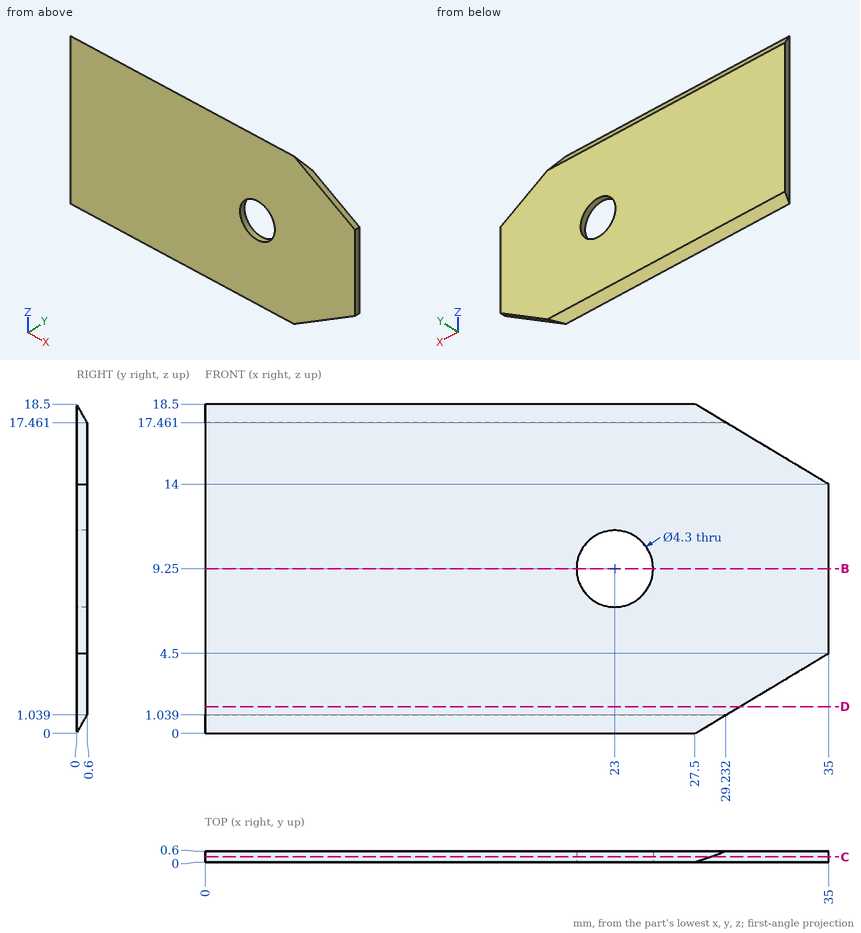
Verification items for this drawing (mm, ordinates from the low corner). Coordinates: 2 decimals unless noted, no trailing zeros. Write each loop counter-clockwise with the first axis right and the second up, starting at its lowest first coordinate (ties: lowest second). Pieces come first, ordered by that corner, then holes. Notation, with made-up numbers: M 17,53 L 66,53 A13 ccw 66,65 Z; hole C -30,-40 d10. An arc over 180 degrees is marked long. Answer as CSV lines item,"result".
Q1. Material ranges on probe 1 along X at (y, z) = (0.2, 9.25); probe 2 along X at (y, z) = (0.4, 10.5); probe 3 along Z at (x, y) = (23, 0.35) (1 decimal), recorded low to high. Write a range as from..to.
Check result:
probe 1,"0..20.85, 25.15..35"
probe 2,"0..21.25, 24.75..35"
probe 3,"0.6..7.1, 11.4..17.9"
Q2. Cross-section at C-C (y = 0.3). Record the boundary of the cut face in (x, z).
Check result:
outline,"M 0,0.52 L 28.37,0.52 L 35,4.5 L 35,14 L 28.37,17.98 L 0,17.98 Z; hole C 23,9.25 d4.3"
Q3. Cross-section at D-D (z = 1.5). Record the boundary of the cut face in (x, y).
Check result:
outline,"M 0,0 L 30,0 L 30,0.6 L 0,0.6 Z"
Q4. Cross-section at B-B (z = 9.25). Record the boundary of the cut face in (x, y).
Check result:
outline,"M 0,0 L 20.85,0 L 20.85,0.6 L 0,0.6 Z; M 25.15,0 L 35,0 L 35,0.6 L 25.15,0.6 Z"
